Model file for the job. Use its own axes, mm. Face numbers are marked on the shaded views. A direction names the side the tool comes from. Coordinates: 2 decimals unless noted, no trailing zeros. Loops run counter-clockwise (first coordinate to the right, second up) from the corner with the lowest first, then second, coordinate; pieces in that order, holes last. Notation, with made-up numbers: M 72.5,-29 L 82.5,-29 A31 ccw 82.5,-2 Z; hole C 60,5.25 d4. An arc over 180 degrees is marked long. Write item = value, one per line. Start each with the question number.
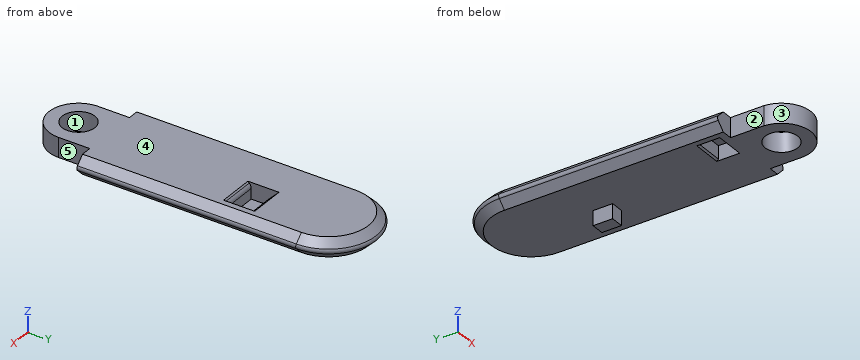
from build123d import *

# Parameters (mm, degrees)
DODANIE_WYCI_GNI_CIE1_DEPTH = 6
SFAZOWANIE1_SIZE            = 3.5
ZAOKR_GLENIE1_R             = 1
SZKIC2_W                    = 11
SZKIC2_H                    = 5.5
WYTNIJ_WYCI_GNI_CIE1_DEPTH  = 5
SZKIC3_W                    = 9
SZKIC3_H                    = 6.5
WYTNIJ_WYCI_GNI_CIE2_DEPTH  = 4.5
SFAZOWANIE2_SIZE            = 0.5
SZKIC4_R                    = 5
DODANIE_WYCI_GNI_CIE2_DEPTH = 6
SZKIC5_W                    = 4
SZKIC5_H                    = 6
DODANIE_WYCI_GNI_CIE3_DEPTH = 4.5
SFAZOWANIE3_SIZE            = 3
SFAZOWANIE4_SIZE            = 1
ZAOKR_GLENIE2_R             = 2


with BuildPart() as part:
    # Szkic1 → Dodanie-wyciągnięcie1 (new body)
    with BuildSketch(Plane.XY):
        with BuildLine():
            ThreePointArc((15.75, 33.5), (0, 49.25), (-15.75, 33.5))
            Line((-15.75, 33.5), (15.75, 33.5))
        make_face()
        with BuildLine():
            Line((15.75, 33.5), (-15.75, 33.5))
            ThreePointArc((-15.75, 33.5), (0, 17.75), (15.75, 33.5))
        make_face()
        with BuildLine():
            ThreePointArc((15.75, 33.5), (0, 17.75), (-15.75, 33.5))
            Line((-15.75, 33.5), (-15.75, -33.5))
            Line((-15.75, -33.5), (15.75, -33.5))
            Line((15.75, -33.5), (15.75, 33.5))
        make_face()
    extrude(amount=-DODANIE_WYCI_GNI_CIE1_DEPTH)

    # Sfazowanie1
    # the kernel refuses this chamfer: 3.5 mm, written as the material it takes off along each edge
    with BuildSketch(Plane(origin=(15.75, -42.500890458, 0), x_dir=(-0.9996219169112968, 0, 0.02749587661058637), z_dir=(0, 1, 0)), Plane(origin=(-15.75, 33.5, 0), x_dir=(0.9996219169112968, 0, 0.02749587661058637), z_dir=(0, -1, 0)), Plane(origin=(-15.75, 33.5, -6), x_dir=(-0.02749587661058661, 0, 0.9996219169112968), z_dir=(0, -1, 0))) as sfazowanie1_piece_1:
        Polygon((SFAZOWANIE1_SIZE * 0.999621916911, -SFAZOWANIE1_SIZE * 0.0274958766106), (-SFAZOWANIE1_SIZE * 0.0274958766106, -SFAZOWANIE1_SIZE * 0.999621916911), (0, 0), align=None)
    extrude(amount=76.000890458, mode=Mode.SUBTRACT)
    with BuildSketch(Plane(origin=(15.75, -42.500890458, -6), x_dir=(-0.9996219169112968, 0, -0.027495876610586358), z_dir=(0, 1, 0))) as sfazowanie1_piece_2:
        Polygon((SFAZOWANIE1_SIZE * 0.999621916911, SFAZOWANIE1_SIZE * 0.0274958766106), (-SFAZOWANIE1_SIZE * 0.0274958766106, SFAZOWANIE1_SIZE * 0.999621916911), (0, 0), align=None)
    extrude(amount=76.000890458, mode=Mode.SUBTRACT)
    with BuildSketch(Plane(origin=(0, 33.5, 0), x_dir=(-1, 0, 0), z_dir=(0, -1, 0))) as sfazowanie1_piece_3:
        Polygon((15.75, SFAZOWANIE1_SIZE), (15.75 - SFAZOWANIE1_SIZE, 0), (15.75, 0), align=None)
    revolve(axis=Axis((0, 33.5, 0), (0, 0, -1)), revolution_arc=180, mode=Mode.SUBTRACT)
    with BuildSketch(Plane(origin=(0, 33.5, -6), x_dir=(1, 0, 0), z_dir=(0, -1, 0))) as sfazowanie1_piece_4:
        Polygon((15.75, SFAZOWANIE1_SIZE), (15.75 - SFAZOWANIE1_SIZE, 0), (15.75, 0), align=None)
    revolve(axis=Axis((0, 33.5, -6), (0, 0, 1)), revolution_arc=180, mode=Mode.SUBTRACT)

    # Zaokrąglenie1
    zaokr_glenie1_edges = [part.edges().sort_by_distance(p)[0] for p in [
        (-15.25, 0, -3),
        (0, 48.75, -3),
        (15.25, 0, -3),
    ]]
    fillet(zaokr_glenie1_edges, radius=ZAOKR_GLENIE1_R)

    # Szkic2 → Wytnij-wyciągnięcie1 (cut)
    with BuildSketch(Plane.XY):
        with Locations((5, 12.25)):
            Rectangle(SZKIC2_W, SZKIC2_H)
    extrude(amount=-WYTNIJ_WYCI_GNI_CIE1_DEPTH, mode=Mode.SUBTRACT)

    # Szkic3 → Wytnij-wyciągnięcie2 (cut)
    with BuildSketch(Plane(origin=(0, 0, -6), x_dir=(-1, 0, 0), z_dir=(0, 0, -1))):
        with Locations((6, -27.988867336)):
            Rectangle(SZKIC3_W, SZKIC3_H)
    extrude(amount=-WYTNIJ_WYCI_GNI_CIE2_DEPTH, mode=Mode.SUBTRACT)

    # Sfazowanie2
    sfazowanie2_edges = [part.edges().sort_by_distance(p)[0] for p in [
        (-6, -24.738867336, -6),
    ]]
    chamfer(sfazowanie2_edges, length=SFAZOWANIE2_SIZE)

    # Szkic4 → Dodanie-wyciągnięcie2 (add)
    with BuildSketch(Plane.XY):
        with BuildLine():
            Line((9, -33.5), (-8.974684649, -33.5))
            Line((-8.974684649, -33.5), (-8.974684649, -43.705386779))
            ThreePointArc((-8.974684649, -43.705386779), (0.337519003, -52.024492564), (9, -43.030823629))
            Line((9, -43.030823629), (9, -33.5))
        make_face()
        with Locations((0, -43.030823629)):
            Circle(SZKIC4_R, mode=Mode.SUBTRACT)
    extrude(amount=-DODANIE_WYCI_GNI_CIE2_DEPTH)

    # Szkic5 → Dodanie-wyciągnięcie3 (add)
    with BuildSketch(Plane(origin=(0, 0, -6), x_dir=(-1, 0, 0), z_dir=(0, 0, -1))):
        with Locations((-2.5, 12)):
            Rectangle(SZKIC5_W, SZKIC5_H)
    extrude(amount=DODANIE_WYCI_GNI_CIE3_DEPTH)

    # Sfazowanie3
    sfazowanie3_edges = [part.edges().sort_by_distance(p)[0] for p in [
        (5, 15, 0),
    ]]
    chamfer(sfazowanie3_edges, length=SFAZOWANIE3_SIZE)

    # Sfazowanie4
    sfazowanie4_edges = [part.edges().sort_by_distance(p)[0] for p in [
        (5, 9.5, 0),
    ]]
    chamfer(sfazowanie4_edges, length=SFAZOWANIE4_SIZE)

    # Zaokrąglenie2
    zaokr_glenie2_edges = [part.edges().sort_by_distance(p)[0] for p in [
        (5, 9.5, -1),
    ]]
    fillet(zaokr_glenie2_edges, radius=ZAOKR_GLENIE2_R)


solid = part.part
Item 1: Probe L1, parallel to Y at x = 0, z = -4.7; L2, parallel to Y at x = 0, z = -1.3; L3, parallel to Z at x = 8.5, y = -9.5. List the from-to ranges inside material, lowest first.
Item 2: Pin check, flat tips, straight feed: pin 1 Ø3 at (y, z) = (-37, -3.5) entering from +X; pin 2 Ø4.5 at (x, z) = (-4, -3) entering from -Y; pin 3 Ø1.6 at (x, y) = (6, 11.5) entering from +Z; pin 4 Ø4 at (x, z) = (10, -8.5) entering from +Y. Stop position of each tip, or through.
Item 3: Cut at B-B (y = 14). Give the cut face in (x, z).
Item 4: Pull direction Y, two halves, no side cores. Call the marked faces 1, 2 and 3: +Y half, -Y half, draft (parallel to the pull), parting line (faces both ways), or undercut.
Item 5: Cut at A-A (y = -12.5). Give the cut face in (x, z), plus the area to 3 significant figures.
Item 6: 3-axis set-ups, long thin cutter, end or side, ignore diameter. For the marked faces 4 and 5: which of +Z, -Z, +X, -X, +Y, -Y reach the whole face in a straight line?
Reported:
q1.L1 = -52.03 to -48.03, -38.03 to 9.5, 15 to 47.05
q1.L2 = -52.03 to -48.03, -38.03 to 9.43, 16.7 to 47.05
q1.L3 = -6 to 0
q2.pin_1 = 9
q2.pin_2 = -51.86
q2.pin_3 = -5
q2.pin_4 = through
q3.outline = M -14.54,-3.71 L -12.25,-6 L 0.5,-6 L 0.5,-10.5 L 4.5,-10.5 L 4.5,-6 L 12.25,-6 L 14.54,-3.71 A1 ccw 14.54,-2.29 L 12.25,0 L 10.5,0 L 10.5,-5 L -0.5,-5 L -0.5,0 L -12.25,0 L -14.54,-2.29 A1 ccw Z
q4.face_1 = undercut
q4.face_2 = draft
q4.face_3 = -Y half
q5.outline = M -14.54,-3.71 L -12.25,-6 L 12.25,-6 L 14.54,-3.71 A1 ccw 14.54,-2.29 L 12.25,0 L -12.25,0 L -14.54,-2.29 A1 ccw Z
q5.area = 165 mm^2
q6.face_4 = +Z, +X, -X, +Y, -Y
q6.face_5 = +Z, -Z, +X, -Y
